Answer from the drawing. Dimensions are ordinates in mm from the lowest x, y and z of the part. A direction names the side the tool comes from. Give positions to 0.01 mm unless a question says otherwise; leave off trailing zeros. Order: outer loops, then holes, each group sorted by start corner. A loop starts at its lowest first (then second) coordinate and runs counter-clockwise, first axis right, second up. Notation, with made-up numbers: M 19.25,-20 L 63.25,-20 A14 cw 63.25,-11 Z; hole C -16.5,-32 d10. An arc over 180 degrees is marked long. One line per item, written item: value.
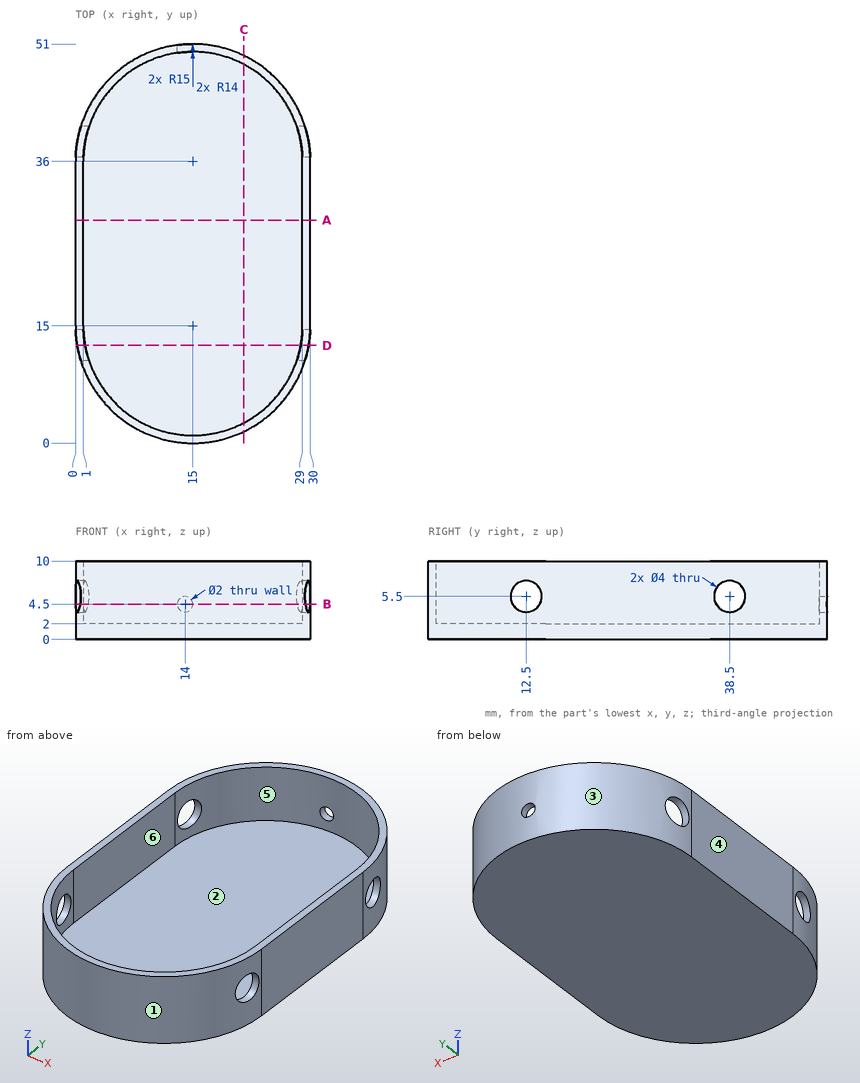
(1) Section A-A, the plane y = 28.5 is taken. Give the vertices of the cut face in (x, z).
Findings:
outline: M 0,0 L 30,0 L 30,10 L 29,10 L 29,2 L 1,2 L 1,10 L 0,10 Z
(2) Which of the six approach directions +Z, -Z, +X, -X, +Y, -Y give full straight-line access (tool end or side, diameter ignored) to the marked faces 1 and 2?
Findings:
face 1: +Z, -Z, -Y
face 2: +Z
(3) Section B-B, the plane z = 4.5 is taken. Give the vertices of the cut face in (x, y), then the cut area to 3 significant figures.
Findings:
outline: M 0,15 A15 ccw 0.02,14.23 L 1.02,14.23 A14 cw 1,15 L 1,36 A14 cw 1.02,36.77 L 0.02,36.77 A15 ccw 0,36 Z; M 0.61,10.77 A15 ccw 29.39,10.77 L 28.35,10.77 A14 cw 1.65,10.77 Z; M 0.61,40.23 L 1.65,40.23 A14 cw 13,49.86 L 13,50.87 A15 ccw Z; M 15,50 A14 cw 28.35,40.23 L 29.39,40.23 A15 ccw 15,51 Z; M 28.98,14.23 L 29.98,14.23 A15 ccw 30,15 L 30,36 A15 ccw 29.98,36.77 L 28.98,36.77 A14 cw 29,36 L 29,15 A14 cw Z
area: 117 mm^2
(4) Given P1, Ø3, axis at x = 11.5, y = 30.5, coming from the +Z side; P2, Ø3, axis at y = 45, z = 8.5, coming from the -X side; P3, Ø3, axis at y = 38.5, z = 5.5, coming from the -X side; P4, Ø5, axis at y = 38.5, z = 5.5, coming from the +X side, each flat-ended and moving along its own axis, determine where each tip first touches the part or whether it passes through.
Findings:
P1: stops at z = 2
P2: stops at x = 2.01
P3: passes through
P4: stops at x = 30
(5) Find the intervals of material crossed by probe 1 along Z at (x, y) = (14, 50.3); probe 2 along X at (y, z) = (30, 3); probe 3 along X at (y, z) = (11, 8.5), in increasing order. Write a range as from..to.
Findings:
probe 1: z = 0..3.5, 5.5..10
probe 2: x = 0..1, 29..30
probe 3: x = 0.54..1.58, 28.42..29.46
(6) Section D-D, the plane y = 12.5 is taken. Give the vertices of the cut face in (x, z), then the cut area to 3 significant figures.
Findings:
outline: M 0.21,0 L 29.79,0 L 29.79,3.5 L 28.77,3.5 L 28.77,2 L 1.23,2 L 1.23,3.5 L 0.21,3.5 Z; M 0.21,7.5 L 1.23,7.5 L 1.23,10 L 0.21,10 Z; M 28.77,7.5 L 29.79,7.5 L 29.79,10 L 28.77,10 Z
area: 67.3 mm^2
(7) Determine the mould class of the marked faces 3, 4, 5 and 6 for opening direction X: pulls with the +X half, pulls with the -X half, needs draft (parallel to the pull), parting line crosses it, or undercut.
Findings:
face 3: parting line crosses it
face 4: pulls with the -X half
face 5: undercut
face 6: undercut
(8) Section C-C, the plane x = 21.5 is taken. Give the vertices of the cut face in (y, z), then the cut area to 3 significant figures.
Findings:
outline: M 1.48,0 L 49.52,0 L 49.52,10 L 48.4,10 L 48.4,2 L 2.6,2 L 2.6,10 L 1.48,10 Z
area: 114 mm^2
